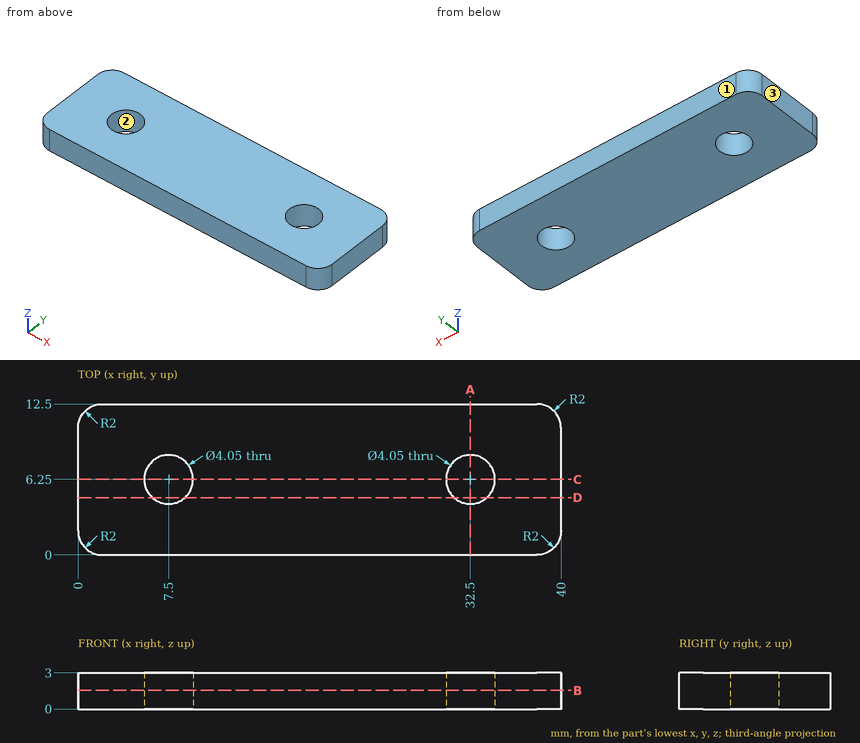
For this review, use the dimensioned drawing (mm, ordinates from the lowest corner) and the shaded views. Round coordinates to 2 decimals unless told otherwise and drop trailing zeros. Order: outer loops, then holes, each group sorted by start corner. A loop starts at its lowest first (then second) coordinate and runs counter-clockwise, first axis right, second up. Notation, with made-up numbers: (25, -6) -> (71, -6) arc R28 cw to (71, 19) -> close; hole circle Ø2 at (6.25, 82). An arc over 180 degrees is marked (long way). One line per item, written item: value. Start each with the question number.
Q1. Take a section at B-B (z = 1.55). Write out the cut boundary in (x, y) (3 decimals), and give its area (3 significant figures).
Q2. Take a section at A-A (x = 32.5). Write out the cut boundary in (y, z) (3 decimals), and give its area (4 significant figures).
Q3. Clearance check with a flat-ended pin moving along its axis: pin 1 Ø6.5 at (x, y) = (32.5, 6.25) entering from -Z. State where the tip first meets the part, or that it passes through.
Q4. Wall thickness on line 1 (Y direction, x = 7.5, z = 2) (3 decimals); line 2 (X direction, y = 4.5, z = 0.8); line 3 (X direction, y = 5.5, z = 2.05): over which ranges is each line inside the solid? List them lowest first.
Q5. Mouldability with a two-part tool opening along X and no side actions: class the marked faces 1, 2 and 3 as released by +X, released by -X, zero draft, split by the parting line, or undercut.
Q6. Take a section at D-D (y = 4.75). Write out the cut boundary in (x, z), and give its area (3 significant figures).
Q7. Take a section at C-C (y = 6.25). Write out the cut boundary in (x, z) (3 decimals).
Reported:
1. outline: (0, 2) arc R2 ccw to (2, 0) -> (38, 0) arc R2 ccw to (40, 2) -> (40, 10.5) arc R2 ccw to (38, 12.5) -> (2, 12.5) arc R2 ccw to (0, 10.5) -> close; hole circle Ø4.05 at (7.5, 6.25); hole circle Ø4.05 at (32.5, 6.25)
1. area: 471 mm2
2. outline: (0, 0) -> (4.225, 0) -> (4.225, 3) -> (0, 3) -> close; (8.275, 0) -> (12.5, 0) -> (12.5, 3) -> (8.275, 3) -> close
2. area: 25.35 mm2
3. pin 1: stops at z = 0
4. line 1: y = 0 to 4.225, 8.275 to 12.5
4. line 2: x = 0 to 6.48, 8.52 to 31.48, 33.52 to 40
4. line 3: x = 0 to 5.62, 9.38 to 30.62, 34.38 to 40
5. face 1: zero draft
5. face 2: undercut
5. face 3: released by -X
6. outline: (0, 0) -> (6.14, 0) -> (6.14, 3) -> (0, 3) -> close; (8.86, 0) -> (31.14, 0) -> (31.14, 3) -> (8.86, 3) -> close; (33.86, 0) -> (40, 0) -> (40, 3) -> (33.86, 3) -> close
6. area: 104 mm2
7. outline: (0, 0) -> (5.475, 0) -> (5.475, 3) -> (0, 3) -> close; (9.525, 0) -> (30.475, 0) -> (30.475, 3) -> (9.525, 3) -> close; (34.525, 0) -> (40, 0) -> (40, 3) -> (34.525, 3) -> close
